Drawing for the job (mm, zero at the part's lowest x, y, z). A direction names the side the tool comes from. Coordinates: 2 decimals unless noted, no trailing zeros. Order: outer loops, then holes, each group sorted by start corner. A loop starts at its lowest first (then second) coordinate and runs counter-clockwise, first axis right, second up. Notation, with made-up numbers: (81, 43) - (127, 43) arc R12 ccw to (127, 65) - close; hole circle Ø9 at (8.5, 31). An arc over 180 degrees is marked (long way). Answer as CSV lines item,"result". Start each with the question number.
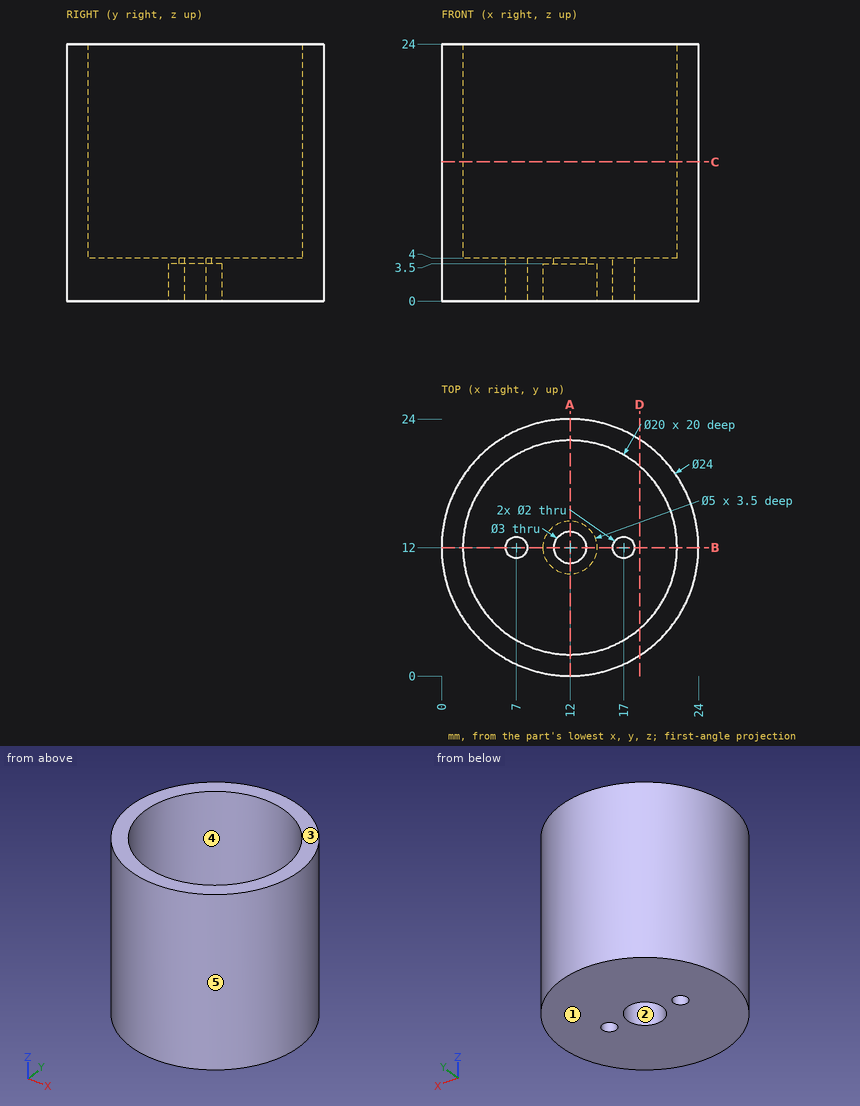
(1) Band-saw the part on A-A on x = 12. List the corners of the cut face in (y, z).
(2) Probe L1, parallel to Z at x = 20.5, y = 10.5; L2, parallel to X at y = 11, z = 20; L3, parallel to Y at x = 12, z = 13.5. List the from-to ranges inside material, lowest first. Write a range as [from, to].
(3) Drop flat-ended pins along their axis: pin 1 Ø2 at (y, z) = (18.5, 6) entering from +X; pin 2 Ø3 at (y, z) = (6.5, 18) entering from -X; pin 3 Ø3 at (x, z) = (19, 8) entering from -Y; pin 4 Ø8 at (y, z) = (10, 21.5) entering from -X. Give the stop position or say it passes through.
(4) Band-saw the part on D-D on x = 18.5. List the corners of the cut face in (y, z), plus the area to 3 significant figures.
(5) Band-saw the part on C-C on z = 13. List the corners of the cut face in (x, y), plus the area to 3 significant figures.
(6) Band-saw the part on B-B on y = 12. List the corners of the cut face in (x, z).
(7) Pull direction Y, two halves, no side cores. Call the marked faces 3, 4 and 5: +Y half, -Y half, draft (parallel to the pull), parting line (faces both ways), or undercut.
(8) Which spindle directions (+Z, -Z, +X, -X, +Y, -Y) get a long thin tool onto all of the face, cutting with end or side? Do the marked faces 1 and 2. Say none if no direction does.
Filled in:
1,outline,"(0, 0) - (9.5, 0) - (9.5, 3.5) - (10.5, 3.5) - (10.5, 4) - (2, 4) - (2, 24) - (0, 24) - close; (13.5, 3.5) - (14.5, 3.5) - (14.5, 0) - (24, 0) - (24, 24) - (22, 24) - (22, 4) - (13.5, 4) - close"
2,L1,"z = [0, 4]"
2,L2,"x = [0.04, 2.05], [21.95, 23.96]"
2,L3,"y = [0, 2], [22, 24]"
3,pin 1,"stops at x = 22.67"
3,pin 2,"stops at x = 0.69"
3,pin 3,"stops at y = 1.33"
3,pin 4,"stops at x = 0"
4,outline,"(1.91, 0) - (22.09, 0) - (22.09, 24) - (19.6, 24) - (19.6, 4) - (4.4, 4) - (4.4, 24) - (1.91, 24) - close"
4,area,"180 mm^2"
5,outline,"circle Ø24 at (12, 12); hole circle Ø20 at (12, 12)"
5,area,"138 mm^2"
6,outline,"(0, 0) - (6, 0) - (6, 4) - (2, 4) - (2, 24) - (0, 24) - close; (8, 0) - (9.5, 0) - (9.5, 3.5) - (10.5, 3.5) - (10.5, 4) - (8, 4) - close; (13.5, 3.5) - (14.5, 3.5) - (14.5, 0) - (16, 0) - (16, 4) - (13.5, 4) - close; (18, 0) - (24, 0) - (24, 24) - (22, 24) - (22, 4) - (18, 4) - close"
7,face 3,"draft"
7,face 4,"undercut"
7,face 5,"parting line"
8,face 1,"-Z, +X, -X, +Y, -Y"
8,face 2,"-Z"
